Verification items for the finished model (mm, model axes). A direction names the side the tool comes from. Round coordinates to 2 decimals unless told otherwise and drop trailing zeros. Loops run counter-clockwise (first coordinate to the right, second up) from the corner with the lowest first, then second, coordinate; pieces in that order, holes last. Notation, with made-up numbers: (44, 12) -> (73, 12) arc R13 cw to (73, 37) -> close; hole circle Ø2 at (4.25, -2.5). An arc over 180 degrees is marked (long way). Use CSV: the item, a comma, the result in double quotes. Start each with the question number.
```python
from build123d import *

# Parameters (mm, degrees)
SKETCH1_W           = 50.8
SKETCH1_H           = 25.4
BOSS_EXTRUDE1_DEPTH = 5.08
SKETCH2_R           = 6.35
BOSS_EXTRUDE2_DEPTH = 6.35
LPATTERN1_COUNT     = 4
LPATTERN1_PITCH     = 12.7
SKETCH2_4_R         = 2.15503395
CUT_EXTRUDE2_DEPTH  = 76.2
SKETCH4_W           = 6.35
SKETCH4_H           = 5.08
CUT_EXTRUDE3_DEPTH  = 5.08
CUT_EXTRUDE4_DEPTH  = 3.81
FILLET1_R           = 2.54


with BuildPart() as part:
    # Sketch1 → Boss-Extrude1 (new body)
    with BuildSketch(Plane(origin=(0, 0, 0), x_dir=(1, 0, 0), z_dir=(0, 1, 0))):
        Rectangle(SKETCH1_W, SKETCH1_H)
    extrude(amount=BOSS_EXTRUDE1_DEPTH)

    # Sketch2 → Boss-Extrude2 (add)
    with BuildSketch(Plane(origin=(25.4, 0, 0), x_dir=(0, 0, -1), z_dir=(1, 0, 0))):
        with Locations((-14.623557735, 6.051646523)):
            Circle(SKETCH2_R)
    boss_extrude2 = extrude(amount=-BOSS_EXTRUDE2_DEPTH)

    # LPattern1: Boss-Extrude2 ×4
    with Locations(*[(-i * LPATTERN1_PITCH, 0, 0) for i in range(1, LPATTERN1_COUNT)]):
        add(boss_extrude2)

    # Sketch2_4 → Cut-Extrude2 (cut)
    with BuildSketch(Plane(origin=(25.4, 0, 0), x_dir=(0, 0, -1), z_dir=(1, 0, 0))):
        with Locations((-14.623557735, 6.051646523)):
            Circle(SKETCH2_4_R)
    extrude(amount=-CUT_EXTRUDE2_DEPTH, mode=Mode.SUBTRACT)

    # Sketch4 → Cut-Extrude3 (cut)
    with BuildSketch(Plane.XY.offset(12.7)):
        with Locations((15.875, 2.54)):
            Rectangle(SKETCH4_W, SKETCH4_H)
        with Locations((3.175, 2.54)):
            Rectangle(SKETCH4_W, SKETCH4_H)
        with Locations((-9.525, 2.54)):
            Rectangle(SKETCH4_W, SKETCH4_H)
        with Locations((-22.225, 2.54)):
            Rectangle(SKETCH4_W, SKETCH4_H)
    extrude(amount=-CUT_EXTRUDE3_DEPTH, mode=Mode.SUBTRACT)

    # Sketch5 → Cut-Extrude4 (cut)
    with BuildSketch(Plane(origin=(0, 5.08, 0), x_dir=(1, 0, 0), z_dir=(0, 1, 0))):
        Polygon((12.7, -7.62), (19.05, -7.62), (19.05, -8.348336382), (25.4, -8.348336382), (25.4, 12.7), (-25.4, 12.7), (-25.4, -7.62), (-19.05, -7.62), (-19.05, -8.348336382), (-12.7, -8.348336382), (-12.7, -7.62), (-6.35, -7.62), (-6.35, -8.348336382), (0, -8.348336382), (0, -7.62), (6.35, -7.62), (6.35, -8.348336382), (12.7, -8.348336382), align=None)
    extrude(amount=-CUT_EXTRUDE4_DEPTH, mode=Mode.SUBTRACT)

    # Fillet1
    fillet1_edges = [part.edges().sort_by_distance(p)[0] for p in [
        (-25.4, 0.635, -12.7),
        (25.4, 0.635, -12.7),
    ]]
    fillet(fillet1_edges, radius=FILLET1_R)


solid = part.part
```
Q1. Release check for a two-part mould opening along X. For faces 6 (the face through (6.35, 3, 14)), 7 (the face through (22.269, 10.355, 19.293)), 8 (the face through (25.4, 4.7, 12.5)) record: +X half, -X half, draft (parallel to the pull), parting line (faces both ways), or undercut.
Q2. Cross-section at C-C (x = -0.5). Record the boundary of the cut face in (y, z).
Q3. Thickness scan on L1, parallel to X at y = 2.25, z = 17.5; L2, parallel to Z at x = 9, y = 6; L3, parallel to Y at x = -10.5, z = 6. Record the ranges inside material, lowest first. Write a range as from..to.
Q4. Cross-section at B-B (y = 7). State how many separate pieces and enclosed holes the cut face has, and give its area (3 significant figures).
Q5. Cross-section at A-A (y = 3.25). Record the boundary of the cut face in (x, z).
Q6. Cross-section at D-D (x = 16). Record the boundary of the cut face in (y, z), and give its area (3 significant figures).
Q7. Tool access check on faces 1 (the face through (-16, 3, 8.348)), 2 (the face through (9.569, 10.355, 19.293)), 3 (the face through (0, 0, 0)), 4 (the face through (-10, 1, 7.62)), 5 (the face through (-22, 1, 7.62)). Record the directions out of +Z, -Z, +X, -X, +Y, -Y that give a thin tool (end or side, any length) a straight path to the whole face; none if there is none.
Q8. Depth check by flat-ended pin: pin 1 Ø1 at (x, y) = (17, 8.5) entering from -Z; pin 2 Ø1 at (x, y) = (-9, 1) entering from +Z; pin 3 Ø1.5 at (x, z) = (7, 4.5) entering from -Y; pin 4 Ø3 at (x, y) = (21, 4) entering from -Z. Enter the tip coordinate at first touch or a pass-through.
Answer list:
1,face 6,"undercut"
1,face 7,"draft"
1,face 8,"+X half"
2,outline,"(0, -12.7) -> (1.27, -12.7) -> (1.27, 8.35) -> (5.08, 8.35) arc R6.35 ccw (long way) to (0, 12.7) -> close; hole circle Ø4.31 at (6.05, 14.62)"
3,L1,"x = -19.05..-12.7, -6.35..0, 6.35..12.7, 19.05..25.4"
3,L2,"z = 8.27..12.47, 16.78..20.97"
3,L3,"y = 0..1.27"
4,separate pieces,"8"
4,enclosed holes,"0"
4,area,"221 mm2"
5,outline,"(-19.05, 8.35) -> (-12.7, 8.35) -> (-12.7, 20.32) -> (-19.05, 20.32) -> close; (-6.35, 8.35) -> (0, 8.35) -> (0, 20.32) -> (-6.35, 20.32) -> close; (6.35, 8.35) -> (12.7, 8.35) -> (12.7, 20.32) -> (6.35, 20.32) -> close; (19.05, 8.35) -> (25.4, 8.35) -> (25.4, 20.32) -> (19.05, 20.32) -> close"
6,outline,"(0, -12.7) -> (1.27, -12.7) -> (1.27, 7.62) -> (0, 7.62) -> close"
6,area,"25.8 mm2"
7,face 1,"-Z, +X, -X"
7,face 2,"+X, -X"
7,face 3,"-Z, +X, -X, -Y"
7,face 4,"+Z, +Y, -Y"
7,face 5,"+Z, -X, +Y, -Y"
8,pin 1,"passes through"
8,pin 2,"stops at z = 7.62"
8,pin 3,"stops at y = 0"
8,pin 4,"stops at z = 8.3"
